Here's how the part is built. I have some questions about the finished solid (model axes, mm). Coordinates: 2 decimals unless noted, no trailing zeros. Write each loop counter-clockwise with the first axis right and the second up, starting at its lowest first coordinate (ties: lowest second). Pieces come first, ordered by that corner, then holes. Notation, with made-up numbers: (76.25, 33) - (112.25, 33) arc R22 ccw to (112.25, 50) - close; hole circle Ø4 at (42, 49.5). An arc over 180 degrees is marked (long way). Answer in a Markdown table with one row per item. Add a question column.
Item 1: If I drill on probe 1 along Z at (x, y) = (-14, 3.2); probe 2 along Z at (x, y) = (18.5, 3.25); probe 3 along X at (y, z) = (2.65, -4), over which ranges is the centre line in solid material (lowest first)? Write a range as from..to.
Item 2: Imagine slicing it at B-B (x = -14.5). Please give me the cut outline in (y, z), plus the area to 3 significant figures.
Item 3: I'm going to push flat-ended pins straight in: pin 1 (3 mm diameter, centred on x = -15.36, z = 8, fed in from -Y); pin 2 (1.5 mm diameter, centred on x = -2, y = 2.5, fed in from -Z). Where does each tip first touch, or does it pass through?
Item 4: We'd pull the mould along Z, two halves only. Please class faces 1 (the face through (3.75, 1.97, -7.84)), 2 (the face through (-13.775, 2.028, 7.792)), 3 (the face through (3.272, 1.972, 7.923)), 4 (the face through (-21.775, 2.028, -0.208)): +Z half, -Z half, draft (parallel to the pull), parting line (faces both ways), or undercut.
Item 5: Imagine slicing it at A-A (z = 0). Please give me the cut outline in (x, y), plus the area to 3 significant figures.
Item 6: Imagine slicing it at C-C (y = 0.75). Please give me the cut outline in (x, z).
Item 7: Imagine slicing it at D-D (z = -5.5). Please give me the cut outline in (x, y).
from build123d import *

# Parameters (mm, degrees)
EXTRUDE_1_DEPTH     = 4
SKETCH_3_R          = 3.1
SKETCH_3_R_2        = 1.6
SKETCH_3_R_3        = 1.65
CUT_EXTRUDE_1_DEPTH = 4


with BuildPart() as part:
    # 草图1 → 凸台-拉伸1 (new body)
    with BuildSketch(Plane(origin=(0, 0, 0), x_dir=(1, 0, 0), z_dir=(0, 1, 0))):
        with BuildLine():
            Line((20.495765525, 4.925982785), (-13.475662945, 10.837162075))
            ThreePointArc((-13.475662945, 10.837162075), (-26.361377172, 4.5e-08), (-13.475663034, -10.837162091))
            Line((-13.475663034, -10.837162091), (20.495765576, -4.925982776))
            ThreePointArc((20.495765576, -4.925982776), (24.638622828, 2.6e-08), (20.495765525, 4.925982785))
        make_face()
    extrude(amount=EXTRUDE_1_DEPTH)

    # 草图3 → 切除-拉伸1 (cut)
    with BuildSketch(Plane(origin=(0, 4, 0), x_dir=(1, 0, 0), z_dir=(0, 1, 0))):
        with Locations(Location((-15.36137507, 8.881e-05, 0), (0, 0, 270))):
            Circle(SKETCH_3_R)
        with Locations(Location((-23.36137507, 8.881e-05, 0), (0, 0, 270))):
            Circle(SKETCH_3_R_2)
        with Locations(Location((-15.36137507, 8.00008881, 0), (0, 0, 270))):
            Circle(SKETCH_3_R_2)
        with Locations(Location((-7.36137507, 8.881e-05, 0), (0, 0, 270))):
            Circle(SKETCH_3_R_2)
        with Locations(Location((-15.36137507, -7.99991119, 0), (0, 0, 270))):
            Circle(SKETCH_3_R_2)
        with Locations(Location((19.638622828, 0, 0), (0, 0, 270))):
            Circle(SKETCH_3_R_3)
    extrude(amount=-CUT_EXTRUDE_1_DEPTH, mode=Mode.SUBTRACT)


solid = part.part
Here are the results:
| question | item | result |
|---|---|---|
| 1 | probe 1 | z = -10.92..-8.84, -7.16..-2.79, 2.78..7.16, 8.84..10.92 |
| 1 | probe 2 | z = -5.27..-1.19, 1.19..5.27 |
| 1 | probe 3 | x = -25.61..22.64 |
| 2 | outline | (0, -10.97) - (4, -10.97) - (4, -9.35) - (0, -9.35) - close; (0, -6.65) - (4, -6.65) - (4, -2.98) - (0, -2.98) - close; (0, 2.98) - (4, 2.98) - (4, 6.65) - (0, 6.65) - close; (0, 9.35) - (4, 9.35) - (4, 10.97) - (0, 10.97) - close |
| 2 | area | 42.3 mm2 |
| 3 | pin 1 | passes through |
| 3 | pin 2 | stops at z = -8.97 |
| 4 | face 1 | -Z half |
| 4 | face 2 | undercut |
| 4 | face 3 | +Z half |
| 4 | face 4 | undercut |
| 5 | outline | (-26.36, 0) - (-24.96, 0) - (-24.96, 4) - (-26.36, 4) - close; (-21.76, 0) - (-18.46, 0) - (-18.46, 4) - (-21.76, 4) - close; (-12.26, 0) - (-8.96, 0) - (-8.96, 4) - (-12.26, 4) - close; (-5.76, 0) - (17.99, 0) - (17.99, 4) - (-5.76, 4) - close; (21.29, 0) - (24.64, 0) - (24.64, 4) - (21.29, 4) - close |
| 5 | area | 140 mm2 |
| 6 | outline | (-13.48, -10.84) - (20.5, -4.93) arc R5 ccw to (20.5, 4.93) - (-13.48, 10.84) arc R11 ccw (long way) to start; hole circle Ø3.2 at (-23.36, 0); hole circle Ø6.2 at (-15.36, 0); hole circle Ø3.2 at (-15.36, -8); hole circle Ø3.2 at (-15.36, 8); hole circle Ø3.2 at (-7.36, 0); hole circle Ø3.3 at (19.64, 0) |
| 7 | outline | (-24.89, 0) - (17.2, 0) - (17.2, 4) - (-24.89, 4) - close |
